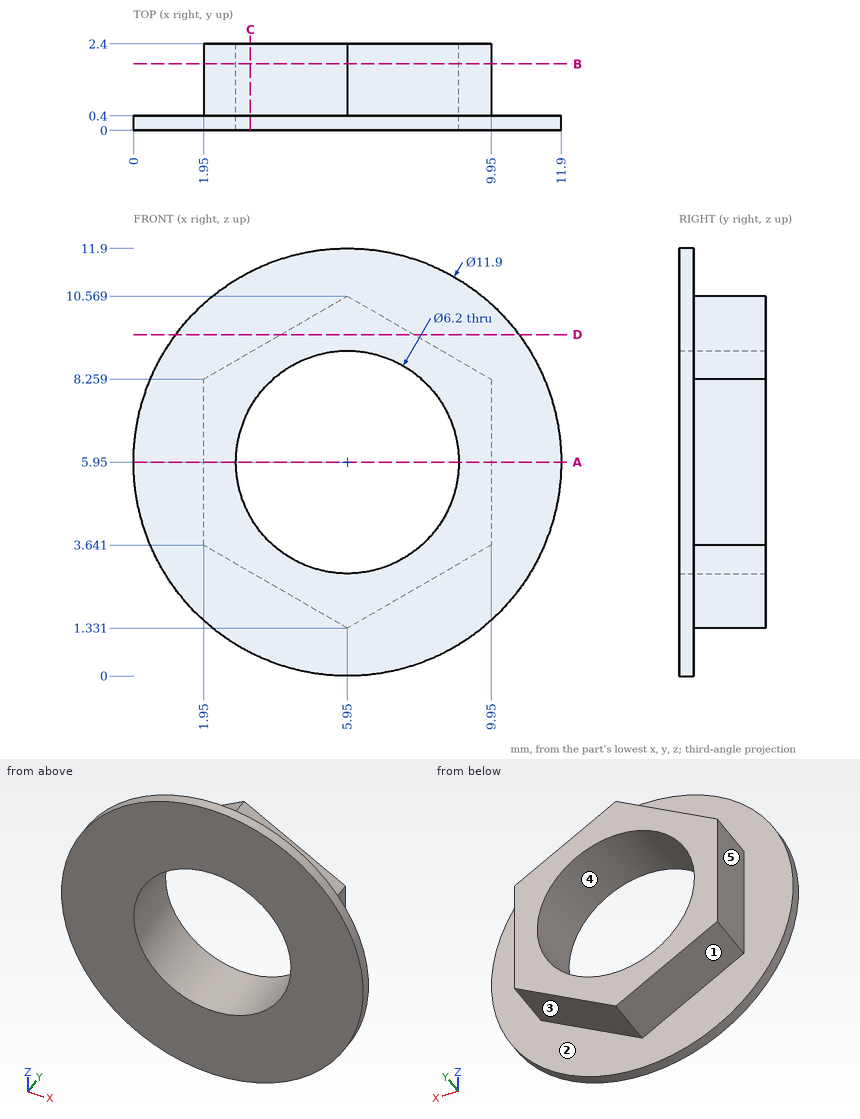
For this review, use the dimensioned drawing (mm, ordinates from the lowest corner) and the shaded views. A direction names the side the tool comes from. Give positions to 0.01 mm unless a question says otherwise; leave off trailing zeros. Order: outer loops, then holes, each group sorted by start corner. A loop starts at its lowest first (then second) coordinate and runs counter-clockwise, first axis right, second up. Notation, with made-up numbers: (6.5, -15.5) - (46.5, -15.5) arc R36 ccw to (46.5, 19.5) - close; hole circle Ø5 at (77, 43.5). An arc over 180 degrees is marked (long way). Use a Markdown table: item, result. Add a question column.
(1) Add section C-C on x = 3.25. Give the boundary of the cut face in (y, z).
(2) Wall thickness on probe 1 along X at (y, z) = (1.25, 5.95); probe 2 along Z at (x, y) = (6.25, 1.1) (1 decimal); probe 3 along Y at (x, z) = (9, 3): over which ranges is each line inside the solid? List them lowest first. Write a range as [from, to].
(3) Add section A-A on z = 5.95. Give the boundary of the cut face in (x, y).
(4) Clearance check with flat-ended pins moving along their axes: P1, Ø1, axis at x = 3.5, y = 1, coming from the -Z side; P2, Ø1, axis at y = 1.5, z = 5.5, coming from the +X side; P3, Ø1, axis at y = 0.5, z = 5, coming from the -X side. State where each tip first meets the part, or that it passes through.
(5) Add section B-B on y = 1.85. Give the boundary of the cut face in (x, z).
(6) Machinability: for the marked faces 1, 2, 3, 4 and 5, which of the approach directions +Z, -Z, +X, -X, +Y, -Y give a long, thin tool a straight path to every point of the face, cutting with its end or side? Answer none if there is none.
(7) Add section D-D on z = 9.5. Give the boundary of the cut face in (x, y) (1 decimal), then the cut area to 3 significant figures.
Report:
| question | item | result |
|---|---|---|
| 1 | outline | (0, 0.65) - (0.4, 0.65) - (0.4, 2.89) - (2.4, 2.89) - (2.4, 4.43) - (0, 4.43) - close; (0, 7.47) - (2.4, 7.47) - (2.4, 9.01) - (0.4, 9.01) - (0.4, 11.25) - (0, 11.25) - close |
| 2 | probe 1 | x = [1.95, 2.85], [9.05, 9.95] |
| 2 | probe 2 | z = [1.5, 2.9], [9, 10.4] |
| 2 | probe 3 | y = [0, 0.4] |
| 3 | outline | (0, 0) - (2.85, 0) - (2.85, 2.4) - (1.95, 2.4) - (1.95, 0.4) - (0, 0.4) - close; (9.05, 0) - (11.9, 0) - (11.9, 0.4) - (9.95, 0.4) - (9.95, 2.4) - (9.05, 2.4) - close |
| 4 | P1 | stops at z = 2.46 |
| 4 | P2 | stops at x = 9.95 |
| 4 | P3 | stops at x = 0.02 |
| 5 | outline | (1.95, 3.64) - (5.95, 1.33) - (9.95, 3.64) - (9.95, 8.26) - (5.95, 10.57) - (1.95, 8.26) - close; hole circle Ø6.2 at (5.95, 5.95) |
| 6 | face 1 | -Z, -X, +Y |
| 6 | face 2 | +Y |
| 6 | face 3 | -Z, +X, +Y |
| 6 | face 4 | +Y, -Y |
| 6 | face 5 | +Z, -Z, -X, +Y |
| 7 | outline | (1.2, 0) - (10.7, 0) - (10.7, 0.4) - (7.8, 0.4) - (7.8, 2.4) - (4.1, 2.4) - (4.1, 0.4) - (1.2, 0.4) - close |
| 7 | area | 11.2 mm² |
